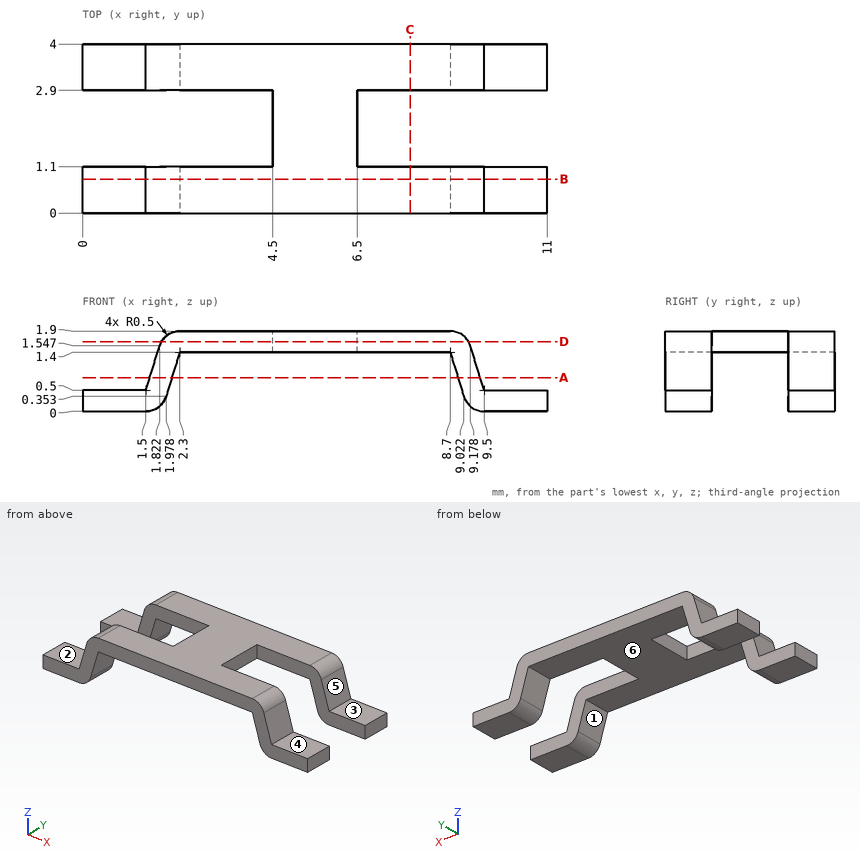
Answer from the drawing. Dimensions are ordinates in mm from the lowest x, y and z of the part. A direction names the side the tool comes from. Coordinates: 2 decimals unless noted, no trailing zeros. Write each loop counter-clockwise with the first axis right and the second up, starting at its lowest first coordinate (ties: lowest second). Pieces come first, ordered by that corner, then holes. Notation, with made-up numbers: (80, 20.25) - (95, 20.25) arc R24 ccw to (95, 41.25) - close; hole circle Ø9 at (-9, 48.5). An arc over 180 degrees is marked (long way). Return JSON: item names as keys, results as strings. Group by question number.
Q1. The part is cut by section D-D on z = 1.65. Write down the section's boundary in (x, y).
Q2. The part is cut by section C-C on x = 7.75. Write down the section's boundary in (y, z).
Q3. Which of the six approach directions +Z, -Z, +X, -X, +Y, -Y give full straight-line access (tool end or side, diameter ignored) to the marked faces 1, 2 and 3?
Q4. A flat-ended cylindrical pin translates along its axis: pin 1 Ø0.6 at (x, y) = (10, 3.5) entering from +Z. Find the tip coordinate at first contact, or state that the pin passes through.
Q5. The part is cut by section B-B on y = 0.8. Write down the section's boundary in (x, z).
Q6. For a pull along X with two mould halves and no side action, classify the marked faces 4, 5 and 6 as +X half, -X half, draft (parallel to the pull), parting line (faces both ways), or undercut.
Q7. Find the intervals of material crossed by line 1 along Z through (x, y) = (10, 0.3); line 2 along Z through (x, y) = (8.25, 3.5); line 3 along X through (y, z) = (0.9, 0.55), in increasing order. Write a range as [from, to].
Q8. The part is cut by section A-A on z = 0.8. Write down the section's boundary in (x, y), and give its area (3 significant figures).
Evaluation:
{
 "1": {"outline": "(1.87, 0) - (9.13, 0) - (9.13, 1.1) - (6.5, 1.1) - (6.5, 2.9) - (9.13, 2.9) - (9.13, 4) - (1.87, 4) - (1.87, 2.9) - (4.5, 2.9) - (4.5, 1.1) - (1.87, 1.1) - close"},
 "2": {"outline": "(0, 1.4) - (1.1, 1.4) - (1.1, 1.9) - (0, 1.9) - close; (2.9, 1.4) - (4, 1.4) - (4, 1.9) - (2.9, 1.9) - close"},
 "3": {"face 1": "-Z, +Y, -Y", "face 2": "+Z, -X, +Y, -Y", "face 3": "+Z, +X, +Y, -Y"},
 "4": {"pin 1": "stops at z = 0.5"},
 "5": {"outline": "(0, 0) - (1.5, 0) arc R0.5 ccw to (1.98, 0.35) - (2.3, 1.4) - (8.7, 1.4) - (9.02, 0.35) arc R0.5 ccw to (9.5, 0) - (11, 0) - (11, 0.5) - (9.5, 0.5) - (9.18, 1.55) arc R0.5 ccw to (8.7, 1.9) - (2.3, 1.9) arc R0.5 ccw to (1.82, 1.55) - (1.5, 0.5) - (0, 0.5) - close"},
 "6": {"face 4": "draft", "face 5": "+X half", "face 6": "undercut"},
 "7": {"line 1": "z = [0, 0.5]", "line 2": "z = [1.4, 1.9]", "line 3": "x = [1.52, 2.04], [8.96, 9.48]"},
 "8": {"outline": "(1.59, 0) - (2.12, 0) - (2.12, 1.1) - (1.59, 1.1) - close; (1.59, 2.9) - (2.12, 2.9) - (2.12, 4) - (1.59, 4) - close; (8.88, 0) - (9.41, 0) - (9.41, 1.1) - (8.88, 1.1) - close; (8.88, 2.9) - (9.41, 2.9) - (9.41, 4) - (8.88, 4) - close", "area": "2.30 mm2"}
}
